Could you check a few things on this model? Use its own coordinates, in mm. A direction names the side the tool comes from. Coordinates: 2 decimals unless noted, no trailing zeros. Write each loop counter-clockwise with the first axis right and the second up, starting at its lowest first coordinate (ties: lowest second). Pieces come first, ordered by that corner, then holes. Notation, with made-up numbers: (50, -28.75) - (97, -28.75) arc R21 cw to (97, 3.25) - close; hole circle Ø11 at (78, 51). An arc over 180 degrees is marked (long way). Answer as a JSON object with one key per item and string values. Group by question number.
1) Will these pins go through, and if not, where does the flat tip stop? pin 1 Ø6 at (x, y) = (7.5, 3) entering from +Z; pin 2 Ø6 at (x, z) = (4, 5) entering from +Y; pin 3 Ø1.5 at (x, y) = (6.5, 1.5) entering from +Z.
2) If we section it at B-B (x = 1.25): Write out the boundary of the cut face in (y, z), plus the area to 3 significant figures.
3) On a 3-axis mill with a long thin cutter (end or side, diameter ignored), from which of +Z, -Z, +X, -X, +Y, -Y can I reach the whole of each face in a straight line? I mean faces 4 (the cylindrical face through (1.96, 4.46, 0.59)), 5 (the cylindrical face through (5.053, 0.676, 2.146)). Say none if no direction works.
4) Please list where these lines run through material, in increasing order: line 1 along Y through (x, z) = (2, 0); line 2 along X through (y, z) = (-5.75, 1.5); line 3 along Y through (x, z) = (1, -1.5).
5) We'd pull the mould along X, two halves only. Please class faces 1 (the flat face through (10.25, -2, -2)), 2 (the cylindrical face through (9.49, -7.81, 1.73)), 3 (the flat face through (0, -2, -2)): released by +X, released by -X, zero draft, split by the parting line, or undercut.
6) If we section it at A-A (x = 9.75): Write out the boundary of the cut face in (y, z), plus the area to 3 significant figures.
```python
from build123d import *

# Parameters (mm, degrees)
SKETCH1_R           = 4.5
BOSS_EXTRUDE1_DEPTH = 10.25
SKETCH3_R           = 2.250000008
CUT_EXTRUDE1_DEPTH  = 34
BOSS_EXTRUDE2_START = -4
SKETCH4_R           = 8
SKETCH4_R_2         = 4.5
BOSS_EXTRUDE2_DEPTH = 4
FILLET1_R           = 2.5
FILLET2_R           = 2.5


with BuildPart() as part:
    # Sketch1 → Boss-Extrude1 (new body)
    with BuildSketch(Plane(origin=(0, 0, 0), x_dir=(0, 0, -1), z_dir=(1, 0, 0))):
        Circle(SKETCH1_R)
    extrude(amount=BOSS_EXTRUDE1_DEPTH)

    # Sketch3 → Cut-Extrude1 (cut)
    with BuildSketch(Plane.ZY):
        Circle(SKETCH3_R)
    extrude(amount=-CUT_EXTRUDE1_DEPTH, mode=Mode.SUBTRACT)

    # Sketch4 → Boss-Extrude2 (add)
    with BuildSketch(Plane(origin=(10.25, 0, 0), x_dir=(0, 0, -1), z_dir=(1, 0, 0)).offset(BOSS_EXTRUDE2_START)):
        Circle(SKETCH4_R)
        Circle(SKETCH4_R_2, mode=Mode.SUBTRACT)
    extrude(amount=BOSS_EXTRUDE2_DEPTH)

    # Fillet1
    fillet1_edges = [part.edges().sort_by_distance(p)[0] for p in [
        (6.25, 0, 8),
    ]]
    fillet(fillet1_edges, radius=FILLET1_R)

    # Fillet2
    fillet2_edges = [part.edges().sort_by_distance(p)[0] for p in [
        (6.25, 0, 4.5),
    ]]
    fillet(fillet2_edges, radius=FILLET2_R)


solid = part.part
```
Here are the results:
{
 "1": {"pin 1": "stops at z = 8", "pin 2": "stops at y = 5.88", "pin 3": "stops at z = 7.37"},
 "2": {"outline": "circle Ø9 at (0, 0); hole circle Ø4.5 at (0, 0)", "area": "47.7 mm²"},
 "3": {"face 4": "-X", "face 5": "+X, -X"},
 "4": {"line 1": "y = -4.5 to -2.25, 2.25 to 4.5", "line 2": "x = 6.25 to 10.25", "line 3": "y = -4.24 to -1.68, 1.68 to 4.24"},
 "5": {"face 1": "released by +X", "face 2": "zero draft", "face 3": "released by -X"},
 "6": {"outline": "circle Ø16 at (0, 0); hole circle Ø4.5 at (0, 0)", "area": "185 mm²"}
}
